```python
from build123d import *

# Parameters (mm, degrees)
SKETCH2_W           = 1500
SKETCH2_H           = 700
BOSS_EXTRUDE1_DEPTH = 30
SKETCH3_W           = 1484
SKETCH3_H           = 690
CUT_EXTRUDE2_DEPTH  = 5
SKETCH9_R           = 19
SKETCH9_R_2         = 20.5
CUT_EXTRUDE3_DEPTH  = 2


with BuildPart() as part:
    # Sketch2 → Boss-Extrude1 (new body)
    with BuildSketch(Plane(origin=(0, 0, 0), x_dir=(1, 0, 0), z_dir=(0, 1, 0))):
        with Locations((447.272601934, 133.030337178)):
            Rectangle(SKETCH2_W, SKETCH2_H)
    extrude(amount=BOSS_EXTRUDE1_DEPTH)

    # Sketch3 → Cut-Extrude2 (cut)
    with BuildSketch(Plane(origin=(0, 30, 0), x_dir=(1, 0, 0), z_dir=(0, 1, 0))):
        with Locations((447.272601934, 133.030337178)):
            Rectangle(SKETCH3_W, SKETCH3_H)
    extrude(amount=-CUT_EXTRUDE2_DEPTH, mode=Mode.SUBTRACT)

    # Sketch9 → Cut-Extrude3 (cut)
    with BuildSketch(Plane(origin=(0, 25, 0), x_dir=(1, 0, 0), z_dir=(0, 1, 0))):
        with Locations(Location((197.272601934, 320.105430206, 0), (0, 0, 270))):
            Circle(SKETCH9_R)
        with Locations(Location((697.300508301, 319.270199385, 0), (0, 0, 270))):
            Circle(SKETCH9_R)
        with Locations(Location((257.272601934, -55.377603043, 0), (0, 0, 270))):
            Circle(SKETCH9_R)
        with Locations(Location((637.272601934, -43.882638763, 0), (0, 0, 270))):
            Circle(SKETCH9_R)
        with Locations(Location((259.572601934, 127.154489334, 0), (0, 0, 270))):
            Circle(SKETCH9_R_2)
        with Locations(Location((634.954920993, 127.154489334, 0), (0, 0, 270))):
            Circle(SKETCH9_R_2)
        with Locations(Location((447.263761463, 12.385030703, 0), (0, 0, 270))):
            Circle(SKETCH9_R_2)
        with Locations(Location((-2.727398066, 320.105430206, 0), (0, 0, 270))):
            Circle(SKETCH9_R)
        with Locations(Location((-2.727398066, -61.969662822, 0), (0, 0, 270))):
            Circle(SKETCH9_R)
        with Locations(Location((897.272601934, 322.611122669, 0), (0, 0, 270))):
            Circle(SKETCH9_R)
        with Locations(Location((897.272601934, -43.882638763, 0), (0, 0, 270))):
            Circle(SKETCH9_R)
    extrude(amount=-CUT_EXTRUDE3_DEPTH, mode=Mode.SUBTRACT)


solid = part.part
```
Input: part model. Units: mm. Frame: model coordinates. A direction names the side the tool comes from. Give positions to 0.01 mm unless a question says otherwise; leave off trailing zeros. Order: outer loops, then holes, each group sorted by start corner. A loop starts at its lowest first (then second) coordinate and runs counter-clockwise, first axis right, second up. Notation, with made-up numbers: (-38.75, 36) - (-5.75, 36) arc R32 cw to (-5.75, 73) - close; hole circle Ø1 at (3.25, 33.25). An arc over 180 degrees is marked (long way). One line per item, written item: value.
1. Line query: probe 1 along Z at (x, y) = (278.5, 25.5); probe 2 along X at (y, z) = (23.5, 72); probe 3 along X at (y, z) = (26.5, -269). Output: solid intervals per line, ascending.
Determined:
probe 1: -483.03 to -478.03, 211.97 to 216.97
probe 2: -302.73 to -18.86, 13.41 to 248.07, 266.48 to 1197.27
probe 3: -302.73 to -294.73, 1189.27 to 1197.27
2. Reachability of faces 1 (the face through (198, 23, -320)), 2 (the face through (437, 15, -483.03)) from +Z, -Z, +X, -X, +Y, -Y: full face, straight path, thin tool, end or side. Return the list, or none.
Determined:
face 1: +Y
face 2: -Z, +X, -X, +Y, -Y
3. Cut plane B-B, the plane x = -52. Output: boundary loops of the cut face in (y, z).
Determined:
outline: (0, -483.03) - (30, -483.03) - (30, -478.03) - (25, -478.03) - (25, 211.97) - (30, 211.97) - (30, 216.97) - (0, 216.97) - close
4. Draft query along Z for faces 3 (the face through (703.01, 24.01, -301.15)), 4 (the face through (437, 0, -138)), 5 (the face through (437, 15, 216.97)), 6 (the face through (638, 23, 44)). Return one class per face: released by +Z, released by -Z, zero draft, split by the parting line, or undercut.
Determined:
face 3: undercut
face 4: zero draft
face 5: released by +Z
face 6: undercut
5. Cut plane A-A, the plane z = 142.5. Output: boundary loops of the cut face in (x, y).
Determined:
outline: (-302.73, 0) - (1197.27, 0) - (1197.27, 30) - (1189.27, 30) - (1189.27, 25) - (-294.73, 25) - (-294.73, 30) - (-302.73, 30) - close
6. Pin query (flat end, axial travel): pin 1 Ø11.5 at (x, z) = (-4.5, 54.5) entering from +Y; pin 2 Ø8 at (x, z) = (-137, -254) entering from +Y. Return the tip coordinate at first contact, or that it passes through.
Determined:
pin 1: y = 23
pin 2: y = 25
